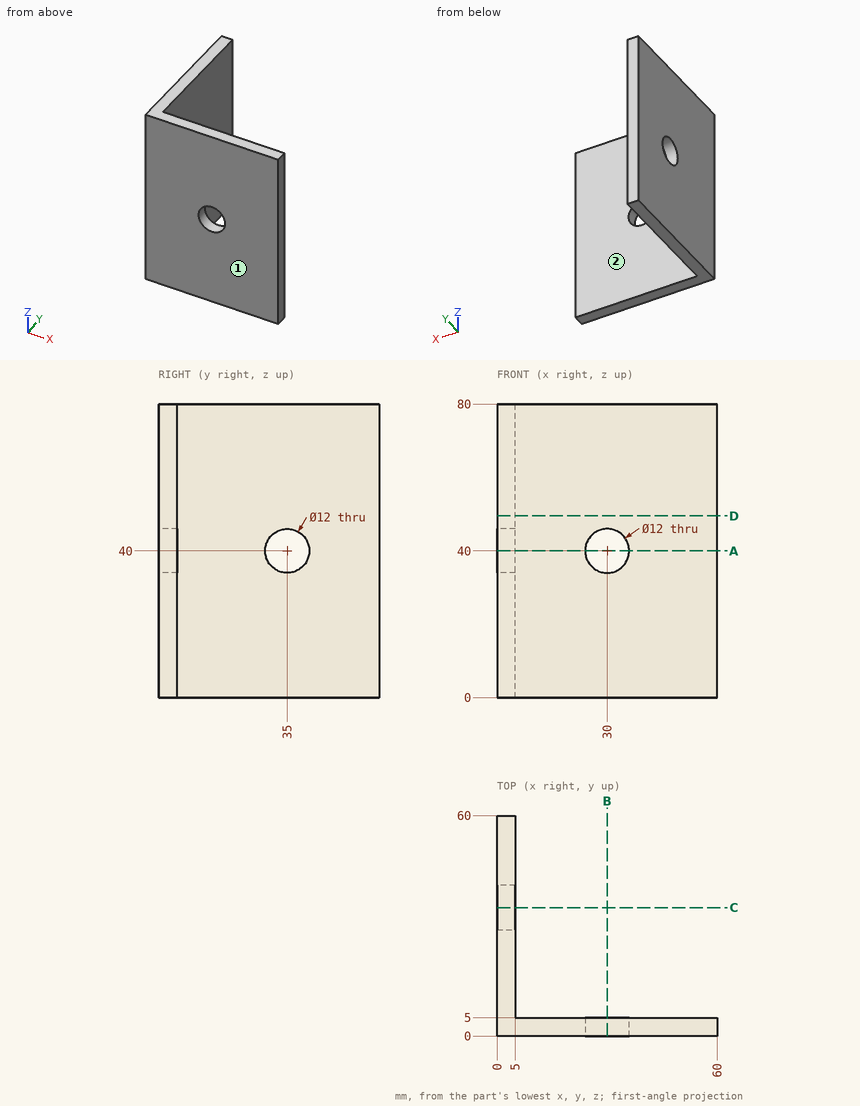
Check sheet for the drawn part. Datum: minimum x, y, z corner. Units: mm. A direction names the side the tool comes from. Coordinates: 2 decimals unless noted, no trailing zeros. Loops run counter-clockwise (first coordinate to the right, second up) from the corner with the lowest first, then second, coordinate; pieces in that order, holes last. Notation, with made-up numbers: (75, 86.25) -> (85, 86.25) arc R17 cw to (85, 104.25) -> close; hole circle Ø1 at (-30.75, 28). An arc over 180 degrees is marked (long way). Answer in a Markdown table with one row per item.
1) Access from +Z, -Z, +X, -X, +Y, -Y to the whole of each face (thin tool, end or side, straight path). Record for the marked faces 1 and 2.
The answers:
| item | result |
|---|---|
| face 1 | +Z, -Z, +X, -X, -Y |
| face 2 | +Z, -Z, +X, +Y |
2) Section check B-B (x = 30). Record the cut outline in (y, z), and give its area (3 significant figures).
The answers:
| item | result |
|---|---|
| outline | (0, 0) -> (5, 0) -> (5, 34) -> (0, 34) -> close; (0, 46) -> (5, 46) -> (5, 80) -> (0, 80) -> close |
| area | 340 mm2 |
3) Section check A-A (z = 40). Record the cut outline in (x, y), and give its area (3 significant figures).
The answers:
| item | result |
|---|---|
| outline | (0, 0) -> (24, 0) -> (24, 5) -> (5, 5) -> (5, 29) -> (0, 29) -> close; (0, 41) -> (5, 41) -> (5, 60) -> (0, 60) -> close; (36, 0) -> (60, 0) -> (60, 5) -> (36, 5) -> close |
| area | 455 mm2 |
4) Depth check by flat-ended pin: P1, Ø3, axis at x = 50, z = 14, coming from the -Y side; P2, Ø12, axis at y = 48, z = 67.5, coming from the +X side; P3, Ø12, axis at x = 38, y = 12.5, coming from the +Z side; P4, Ø6, axis at x = 42, z = 52.5, coming from the +Y side. Enter the tip coordinate at first touch or a pass-through.
The answers:
| item | result |
|---|---|
| P1 | stops at y = 0 |
| P2 | stops at x = 5 |
| P3 | passes through |
| P4 | stops at y = 5 |
5) Section check D-D (z = 49.5). Record the cut outline in (x, y).
The answers:
| item | result |
|---|---|
| outline | (0, 0) -> (60, 0) -> (60, 5) -> (5, 5) -> (5, 60) -> (0, 60) -> close |
6) Scan lines: line 1 along Z through (x, y) = (30, 2.3); line 2 along X through (y, z) = (36, 61). Record each from-to range of solid material in increasing order. Write a range as from..to.
The answers:
| item | result |
|---|---|
| line 1 | z = 0..34, 46..80 |
| line 2 | x = 0..5 |
